Part model, mm, in its own coordinate system. A direction names the side the tool comes from. Give positions to 0.01 mm unless a question says otherwise; leave off trailing zeros. Loops run counter-clockwise (first coordinate to the right, second up) from the corner with the lowest first, then second, coordinate; pieces in that order, holes last. Notation, with made-up numbers: M 24,-14.5 L 72,-14.5 A13 cw 72,-5.5 Z; hole C 23,42.25 d1. An arc over 180 degrees is marked long. Answer in a Markdown table with one row per item.
Autodesk Inventor part; units mm, degrees
ref_plane "YZ Plane" through (0, 0, 0) normal (1, 0, 0) x (0, 1, 0)
ref_plane "XY Plane" through (0, 0, 0) normal (0, 0, 1) x (1, 0, 0)
sketch "Sketch1" plane through (0, 0, 0) normal (0, 0, 1) x (1, 0, 0)
  circle A0 centre (0, 0) radius 5.08
  dimension "d0" = 10.16
extrude "Extrusion1" add sketch "Sketch1" along normal blind 12.954
sketch "Sketch2" plane through (0, 0, 12.954) normal (0, 0, 1) x (1, 0, 0)
  circle A0 centre (0, 0) radius 3.683
  dimension "d3" = 7.366
extrude "Extrusion2" add sketch "Sketch2" along normal blind 9.398
sketch "Sketch4" plane through (0, 0, 22.352) normal (0, 0, 1) x (1, 0, 0)
  circle A0 centre (0, 0) radius 2.413
  dimension "d9" = 4.826
extrude "Extrusion3" cut sketch "Sketch4" against normal blind 9.652
sketch "Sketch5" plane through (0, 0, 22.352) normal (0, 0, 1) x (1, 0, 0)
  circle A0 centre (0, 0) radius 3.175
  dimension "d12" = 6.35
extrude "Extrusion4" cut sketch "Sketch5" against normal blind 1.27
sketch "Sketch6" plane through (0, 0, 0) normal (0, 0, -1) x (-1, 0, 0)
  circle A0 centre (0, 0) radius 2.413
  dimension "d15" = 4.826
extrude "Extrusion5" cut sketch "Sketch6" against normal blind 11.176
sketch "Sketch7" plane through (0, 0, 0) normal (0, 0, -1) x (-1, 0, 0)
  circle A0 centre (0, 0) radius 3.175
  dimension "d18" = 6.35
extrude "Extrusion6" cut sketch "Sketch7" against normal blind 6.35
sketch "Sketch8" plane through (0, 0, 0) normal (0, 0, -1) x (-1, 0, 0)
  circle A0 centre (0, 0) radius 3.683
  circle A1 centre (0, 0) radius 5.2614
  dimension "d21" = 7.366
extrude "Extrusion7" cut sketch "Sketch8" against normal blind 11.176
sketch "Sketch9" plane through (0, 0, 0) normal (0, 0, -1) x (-1, 0, 0)
  circle A0 centre (0, 0) radius 3.81
  dimension "d24" = 7.62
extrude "Extrusion8" add sketch "Sketch9" against normal blind 1.27
sketch "Sketch10" plane through (0, 0, 0) normal (0, 0, -1) x (-1, 0, 0)
  circle A0 centre (0, 0) radius 3.175
extrude "Extrusion9" cut sketch "Sketch10" against normal blind 1.27
ref_plane "Work Plane1" through (0, 5.08, 0) normal (0, 1, 0) x (-1, 0, 0)
sketch "Sketch13" plane through (0, 5.08, 0) normal (0, 1, 0) x (-1, 0, 0)
  line L0 (0, 0) -> (-0.508, 0)
  line L1 (-0.508, 0) -> (-0.508, 5.08)
  line L2 (-0.508, 5.08) -> (0, 5.08)
  line L3 (0, 5.08) -> (0, 0)
  line L4 (0, 0) -> (0.508, 0)
  line L5 (0.508, 0) -> (0.508, 5.08)
  line L6 (0.508, 5.08) -> (0, 5.08)
  line L7 (0, 5.08) -> (0, 0)
  dimension "d30" = 5.08
  dimension "d31" = 0.508
  dimension "d32" = 0.508
  dimension "d33" = 5.08
extrude "Extrusion10" cut sketch "Sketch13" against normal blind 10.16
properties part number "axle"
(1) Pin check, flat tips, straight feed: pin 1 Ø3 at (x, y) = (0, 0) entering from +Z; pin 2 Ø5 at (x, y) = (0, 0) entering from -Z; pin 3 Ø2 at (y, z) = (-3.5, 17.5) entering from -X. Stop position of each tip, or through.
Recorded:
| item | result |
|---|---|
| pin 1 | stops at z = 12.7 |
| pin 2 | stops at z = 6.35 |
| pin 3 | stops at x = -2.7 |
(2) Drill centre lines: line 1 along Y through (x, z) = (0, 15.75); line 2 along Z through (x, y) = (3, -2.5); line 3 along Y through (x, z) = (0.75, 7.25). Where is each one in solid material? Low to high.
Recorded:
| item | result |
|---|---|
| line 1 | y = -3.68 to -2.41, 2.41 to 3.68 |
| line 2 | z = 11.18 to 12.95 |
| line 3 | y = -3.61 to -2.29, 2.29 to 3.61 |
(3) Pull direction X, two halves, no side cores. Call faces 4 (the face through (1.915, -1.468, 8.729)), 5 (the face through (3, 3, 12.954)), 6 (the face through (3.81, 0.08, 0.63)), 7 (the face through (-1.915, -1.468, 16.95)): +X half, -X half, draft (parallel to the pull), parting line (faces both ways), or undercut.
Recorded:
| item | result |
|---|---|
| face 4 | undercut |
| face 5 | draft |
| face 6 | +X half |
| face 7 | undercut |
(4) Saw through at D-D (z = 18.25). Write the cut outline in (x, y).
Recorded:
| item | result |
|---|---|
| outline | C 0,0 d7.37; hole C 0,0 d4.83 |
(5) Saw through at C-C (z = 4). Write the cut outline in (x, y) (3 decimals).
Recorded:
| item | result |
|---|---|
| outline | M -0.508,-3.648 L -0.508,-3.134 A3.175 cw -0.508,3.134 L -0.508,3.648 A3.683 ccw Z; M 0.508,-3.648 A3.683 ccw 0.508,3.648 L 0.508,3.134 A3.175 cw 0.508,-3.134 Z |
(6) Saw through at B-B (x = 0). Write the cut outline in (y, z) (3 decimals).
Recorded:
| item | result |
|---|---|
| outline | M -5.08,11.176 L -3.683,11.176 L -3.683,5.08 L -3.175,5.08 L -3.175,6.35 L -2.413,6.35 L -2.413,11.176 L 2.413,11.176 L 2.413,6.35 L 3.175,6.35 L 3.175,5.08 L 3.683,5.08 L 3.683,11.176 L 5.08,11.176 L 5.08,12.954 L 3.683,12.954 L 3.683,22.352 L 3.175,22.352 L 3.175,21.082 L 2.413,21.082 L 2.413,12.7 L -2.413,12.7 L -2.413,21.082 L -3.175,21.082 L -3.175,22.352 L -3.683,22.352 L -3.683,12.954 L -5.08,12.954 Z |
(7) Which spindle directions (+Z, -Z, +X, -X, +Y, -Y) get a long thin tool onto all of the face, cutting with end or side? Do faces 1 (the face through (-3.3, -0.5, 0)), 2 (the face through (1.699, 3.267, 17.587)), 3 (the face through (0, 0, 11.176)). Say none if no direction does.
Recorded:
| item | result |
|---|---|
| face 1 | -Z, +X, -X, +Y, -Y |
| face 2 | +Z |
| face 3 | -Z |
